from build123d import *

# Parameters (mm, degrees)
SKETCH1_W                       = 93.98
SKETCH1_H                       = 55.88
SKETCH1_R                       = 1.905
BOSS_EXTRUDE1_DEPTH             = 3.81
F_7_64_0_10938_DIAMETER_HOLE1_D = 2.778252
FILLET1_R                       = 2.54
EXTRUDE_THIN1_DEPTH             = 3.81
FILLET2_R                       = 1.27
FILLET3_R                       = 0.635


with BuildPart() as part:
    # Sketch1 → Boss-Extrude1 (new body)
    with BuildSketch(Plane(origin=(0, 0, 0), x_dir=(1, 0, 0), z_dir=(0, 1, 0))):
        Rectangle(SKETCH1_W, SKETCH1_H)
        with Locations(Location((0, 0, 0), (0, 0, 90))):
            Circle(SKETCH1_R, mode=Mode.SUBTRACT)
        with BuildLine():
            Line((40.073298182, 19.676259764), (38.726259764, 21.023298182))
            ThreePointArc((38.726259764, 21.023298182), (38.726259764, 23.896980141), (41.599941723, 23.896980141))
            Line((41.599941723, 23.896980141), (42.946980141, 22.549941723))
            ThreePointArc((42.946980141, 22.549941723), (42.946980141, 19.676259764), (40.073298182, 19.676259764))
        make_face(mode=Mode.SUBTRACT)
        with BuildLine():
            Line((-40.073298182, 19.676259764), (-38.726259764, 21.023298182))
            ThreePointArc((-38.726259764, 21.023298182), (-38.726259764, 23.896980141), (-41.599941723, 23.896980141))
            Line((-41.599941723, 23.896980141), (-42.946980141, 22.549941723))
            ThreePointArc((-42.946980141, 22.549941723), (-42.946980141, 19.676259764), (-40.073298182, 19.676259764))
        make_face(mode=Mode.SUBTRACT)
        with BuildLine():
            Line((40.073298182, -19.676259764), (38.726259764, -21.023298182))
            ThreePointArc((38.726259764, -21.023298182), (38.726259764, -23.896980141), (41.599941723, -23.896980141))
            Line((41.599941723, -23.896980141), (42.946980141, -22.549941723))
            ThreePointArc((42.946980141, -22.549941723), (42.946980141, -19.676259764), (40.073298182, -19.676259764))
        make_face(mode=Mode.SUBTRACT)
        with BuildLine():
            Line((-40.073298182, -19.676259764), (-38.726259764, -21.023298182))
            ThreePointArc((-38.726259764, -21.023298182), (-38.726259764, -23.896980141), (-41.599941723, -23.896980141))
            Line((-41.599941723, -23.896980141), (-42.946980141, -22.549941723))
            ThreePointArc((-42.946980141, -22.549941723), (-42.946980141, -19.676259764), (-40.073298182, -19.676259764))
        make_face(mode=Mode.SUBTRACT)
    extrude(amount=BOSS_EXTRUDE1_DEPTH)

    # 7/64 (0.10938) Diameter Hole1 (through all)
    with Locations(Plane(origin=(0, 0, 0), x_dir=(-1, 0, 0), z_dir=(0, -1, 0))):
        with Locations((-18.6309, 0), (0, 7.112), (-7.112, 0), (7.112, 0), (18.6309, 0), (0, -7.112)):
            Hole(F_7_64_0_10938_DIAMETER_HOLE1_D / 2)

    # Fillet1
    fillet1_edges = [part.edges().sort_by_distance(p)[0] for p in [
        (-46.99, 1.905, 27.94),
        (46.99, 1.905, 27.94),
        (46.99, 1.905, -27.94),
        (-46.99, 1.905, -27.94),
    ]]
    fillet(fillet1_edges, radius=FILLET1_R)

    # Sketch4 → Extrude-Thin1 (add)
    with BuildSketch(Plane(origin=(0, 0, 0), x_dir=(1, 0, 0), z_dir=(0, 1, 0))):
        with BuildLine():
            Line((-40.64, 10.16), (-40.64, -10.16))
            ThreePointArc((-40.64, -10.16), (-36.920256121, -19.140256121), (-27.94, -22.86))
            Line((-27.94, -22.86), (27.94, -22.86))
            ThreePointArc((27.94, -22.86), (36.920256121, -19.140256121), (40.64, -10.16))
            Line((40.64, -10.16), (40.64, 10.16))
            ThreePointArc((40.64, 10.16), (36.920256121, 19.140256121), (27.94, 22.86))
            Line((27.94, 22.86), (-27.94, 22.86))
            ThreePointArc((-27.94, 22.86), (-36.920256121, 19.140256121), (-40.64, 10.16))
        make_face()
        with BuildLine():
            Line((-36.83, 10.16), (-36.83, -10.16))
            ThreePointArc((-36.83, -10.16), (-34.226179285, -16.446179285), (-27.94, -19.05))
            Line((-27.94, -19.05), (27.94, -19.05))
            ThreePointArc((27.94, -19.05), (34.226179285, -16.446179285), (36.83, -10.16))
            Line((36.83, -10.16), (36.83, 10.16))
            ThreePointArc((36.83, 10.16), (34.226179285, 16.446179285), (27.94, 19.05))
            Line((27.94, 19.05), (-27.94, 19.05))
            ThreePointArc((-27.94, 19.05), (-34.226179285, 16.446179285), (-36.83, 10.16))
        make_face(mode=Mode.SUBTRACT)
    extrude(amount=-EXTRUDE_THIN1_DEPTH)

    # Fillet2
    fillet2_edges = [part.edges().sort_by_distance(p)[0] for p in [
        (-36.920256121, -3.81, 19.140256121),
        (-40.64, -3.81, 0),
        (-36.920256121, -3.81, -19.140256121),
        (0, -3.81, -22.86),
        (36.920256121, -3.81, -19.140256121),
        (40.64, -3.81, 0),
        (36.920256121, -3.81, 19.140256121),
        (0, -3.81, 22.86),
        (-36.83, -3.81, 0),
        (-34.226179285, -3.81, 16.446179285),
        (0, -3.81, 19.05),
        (34.226179285, -3.81, 16.446179285),
        (36.83, -3.81, 0),
        (34.226179285, -3.81, -16.446179285),
        (0, -3.81, -19.05),
        (-34.226179285, -3.81, -16.446179285),
    ]]
    fillet(fillet2_edges, radius=FILLET2_R)

    # Fillet3
    fillet3_edges = [part.edges().sort_by_distance(p)[0] for p in [
        (-46.99, 0, 0),
        (0, 0, -27.94),
        (46.99, 0, 0),
        (0, 0, 27.94),
        (46.246051224, 0, 27.196051224),
        (46.246051224, 0, -27.196051224),
        (-46.246051224, 0, 27.196051224),
        (-46.246051224, 0, -27.196051224),
        (-36.920256121, 0, 19.140256121),
        (0, 0, 22.86),
        (36.920256121, 0, 19.140256121),
        (40.64, 0, 0),
        (36.920256121, 0, -19.140256121),
        (0, 0, -22.86),
        (-36.920256121, 0, -19.140256121),
        (-40.64, 0, 0),
    ]]
    fillet(fillet3_edges, radius=FILLET3_R)


solid = part.part
Model file for the job. Use its own axes, mm. A direction names the side the tool comes from. Give positions to 0.01 mm unless a question says otherwise; leave off trailing zeros. Use a Markdown table: item, result. Add a question column.
(1) Mould opens along X. For faces 1 (the cylindrical face through (37.02, -1.57, -19.04)), 2 (the flat face through (0, -1, -19.05)), 3 (the cylindrical face through (-0.181, 1.932, 5.735)), 4 (the cylindrical face through (-46.266, 2.245, -27.176)) say: +X half, -X half, draft (parallel to the pull), parting line (faces both ways), or undercut.
(2) Drop flat-ended pins along their axis: pin 1 Ø3 at (x, z) = (3.5, -11.5) entering from -Y; pin 2 Ø1.5 at (y, z) = (-1.5, 2.5) entering from -X; pin 3 Ø1.5 at (x, y) = (-0.5, -1.5) entering from -Z. Give the stop position or say it passes through.
(3) Wall check: line 1 along Z through (x, y) = (42, 0.5); line 2 along X through (y, z) = (2.5, -21); line 3 along Y through (x, z) = (-21.5, 12). Give the ranges that are in metal, low to high.
(4) Tool access for faces 5 (the flat face through (46.99, 2, 0)), 6 (the cylindrical face through (36.82, -1.57, 19.24)), 7 (the flat face through (0, -1, 19.05)): list every direction of +Z, -Z, +X, -X, +Y, -Y with a clear straight run to the whole face (end or side of a thin tool).
(5) Slice it at A-A on x = 0. Give the number of separate pieces and of enclosed holes in the cut face, and give its area (3 significant figures).
Filled sheet:
| question | item | result |
|---|---|---|
| 1 | face 1 | +X half |
| 1 | face 2 | undercut |
| 1 | face 3 | undercut |
| 1 | face 4 | -X half |
| 2 | pin 1 | y = 0 |
| 2 | pin 2 | x = -40.64 |
| 2 | pin 3 | z = -22.86 |
| 3 | line 1 | -27.93 to -23.5, -19.14 to 19.14, 23.5 to 27.93 |
| 3 | line 2 | -46.99 to -43.54, -38.75 to 38.75, 43.54 to 46.99 |
| 3 | line 3 | 0 to 3.81 |
| 4 | face 5 | +Z, -Z, +X, +Y, -Y |
| 4 | face 6 | +Z, +X, -Y |
| 4 | face 7 | -Y |
| 5 | separate pieces | 4 |
| 5 | enclosed holes | 0 |
| 5 | area | 205 mm2 |
